```python
from build123d import *

# Parameters (mm, degrees)
F1_DEPTH = 2
F2_DEPTH = 6
F3_R     = 4.99999
F4_R     = 1


# Not quite as in the source:
# - a fillet or chamfer is up to 0.001 mm smaller than in the source, because OpenCascade refuses the exact size


with BuildPart() as f1:
    # F0 (on Top) → F1 (new body)
    with BuildSketch(Plane.XY):
        Polygon((5, 70), (0, 70), (-5, 70), (-5, 5), (-70, 5), (-70, -5), (-5, -5), (-5, -70), (0, -70), (5, -70), (5, -5), (70, -5), (70, 5), (5, 5), align=None)
    extrude(amount=F1_DEPTH)

    # F0 (on Top) → F2 (join)
    with BuildSketch(Plane.XY):
        Polygon((0, 72.5), (-7.5, 72.5), (-7.5, 7.5), (-72.5, 7.5), (-72.5, 6.8834697455), (-72.5, -7.5), (-7.5, -7.5), (-7.5, -72.5), (0, -72.5), (7.5, -72.5), (7.5, -7.5), (72.5, -7.5), (72.5, 7.5), (7.5, 7.5), (7.5, 72.5), align=None)
        Polygon((-5, 70), (0, 70), (5, 70), (5, 5), (70, 5), (70, -5), (5, -5), (5, -70), (0, -70), (-5, -70), (-5, -5), (-70, -5), (-70, 5), (-5, 5), align=None, mode=Mode.SUBTRACT)
    extrude(amount=F2_DEPTH)

    # F3 (radius 5 in the source; OpenCascade refuses exactly that, so slightly less here)
    f3_edges = [f1.edges().sort_by_distance(p)[0] for p in [
        (-5, 70, 4),
        (-70, 5, 4),
        (5, 70, 4),
        (70, 5, 4),
        (70, -5, 4),
        (5, -70, 4),
        (-70, -5, 4),
        (-5, -70, 4),
        (-7.5, 72.5, 3),
        (7.5, 72.5, 3),
        (72.5, 7.5, 3),
        (72.5, -7.5, 3),
        (7.5, -72.5, 3),
        (-72.5, 7.5, 3),
        (-72.5, -7.5, 3),
        (-7.5, -72.5, 3),
        (-7.5, -7.5, 3),
        (-5, 5, 4),
        (5, 5, 4),
        (5, -5, 4),
        (-7.5, 7.5, 3),
        (-5, -5, 4),
        (7.5, 7.5, 3),
        (7.5, -7.5, 3),
    ]]
    fillet(f3_edges, radius=F3_R)

    # F4
    f4_edges = [f1.edges().sort_by_distance(p)[0] for p in [
        (7.5, 40, 0),
    ]]
    fillet(f4_edges, radius=F4_R)


solid = f1.part
```
Read the model definition and answer for the solid it produces. Units are mm, in the model's axes. A direction names the side the tool comes from. Round coordinates to 2 decimals unless told otherwise and drop trailing zeros. Write each loop counter-clockwise with the first axis right and the second up, starting at its lowest first coordinate (ties: lowest second). Pieces come first, ordered by that corner, then holes. Notation, with made-up numbers: (1.25, 82) - (26.25, 82) arc R14 cw to (26.25, 93) - close; hole circle Ø6 at (46.5, 62). An arc over 180 degrees is marked (long way). Use CSV: the item, a comma, the result in double quotes.
Q1. A tool of negligible diameter and unlimited length cuts with its end or side. For faces 1 (the cylindrical face through (-6, -7, 4)), 2 (the cylindrical face through (6, -71.07, 3.53)), from which of +Z, -Z, +X, -X, +Y, -Y can it reach the whole face along a straight path? Write none if from no direction.
Values:
face 1,"+Z"
face 2,"+Z, -Z, +X, -Y"
Q2. Straight lines are drawn through the part: line 1 along Y through (x, z) = (-14.5, 3.55); line 2 along Y through (x, z) = (-38, 1.35). For each, find the intervals that lie inside material, in ascending order.
Values:
line 1,"y = -7.5 to -5, 5 to 7.5"
line 2,"y = -7.5 to 7.5"
Q3. Each of these flat-tipped pins is pushed along its axis until it touches: pin 1 Ø3 at (x, z) = (47, 4) entering from -Y; pin 2 Ø3 at (x, z) = (-27.5, 1.5) entering from +Y; pin 3 Ø5 at (x, y) = (40, 2) entering from +Z. Where does it stop, or does it pass through?
Values:
pin 1,"stops at y = -7.5"
pin 2,"stops at y = 7.5"
pin 3,"stops at z = 2"
Q4. Determine the mould class of faces 3 (the flat face through (0, 72.5, 3)), 4 (the flat face through (5, 38, 4)), 5 (the flat face through (-7.5, -40, 3)), 6 (the cylindrical face through (69, -3, 4)) for opening direction X: +X half, -X half, draft (parallel to the pull), parting line (faces both ways), or undercut.
Values:
face 3,"draft"
face 4,"undercut"
face 5,"-X half"
face 6,"undercut"
Q5. Find section A-A, the plane y = -22.5. Write down the section's boundary in (x, z), then the cut area to 3 significant figures.
Values:
outline,"(-7.5, 1) arc R1 ccw to (-6.5, 0) - (6.5, 0) arc R1 ccw to (7.5, 1) - (7.5, 6) - (5, 6) - (5, 2) - (-5, 2) - (-5, 6) - (-7.5, 6) - close"
area,"49.6 mm²"
